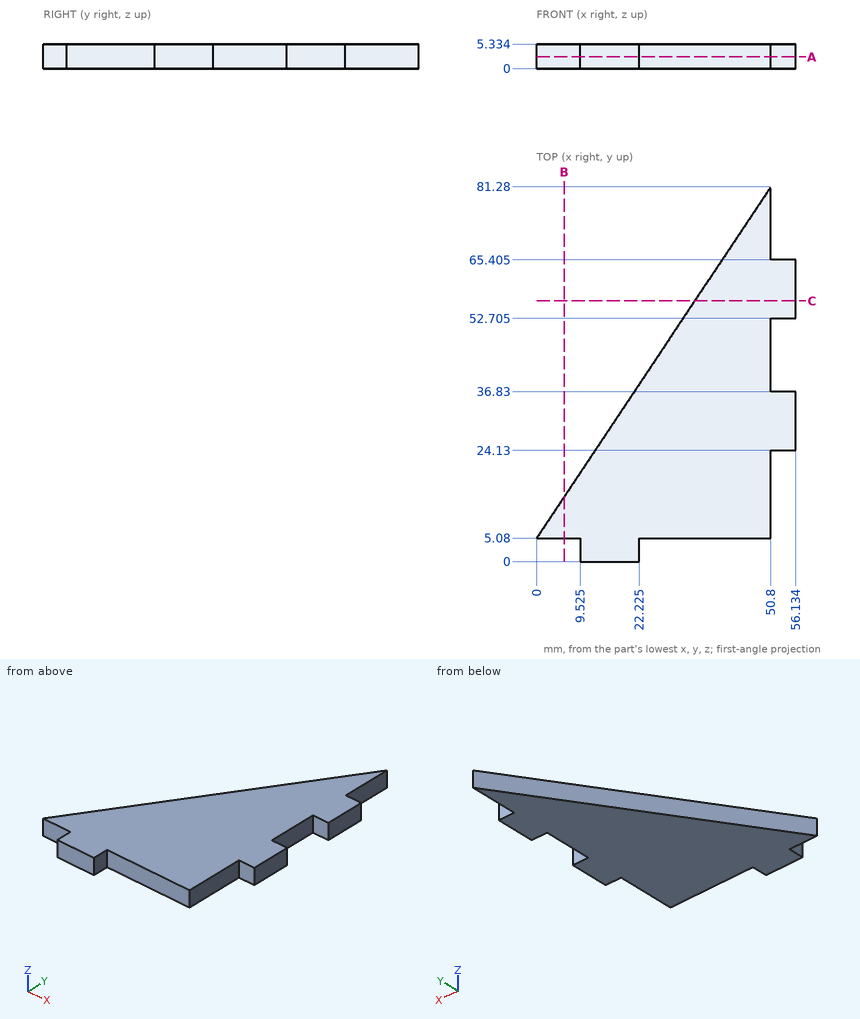
The drawing under review shows one solid part. Ordinate dimensions are in mm from its lowest x, y, z. Give positions to 0.01 mm unless a question says otherwise; leave off trailing zeros. Loops run counter-clockwise (first coordinate to the right, second up) from the corner with the lowest first, then second, coordinate; pieces in that order, holes last. Notation, with made-up numbers: M 83,23 L 101,23 A23 cw 101,33 Z; hole C 79,-2 d7. An arc over 180 degrees is marked long. One line per item, written item: value. Start each with the question number.
Q1. Add section B-B (x = 6). Give the boundary of the cut face in (y, z).
Q2. Add section C-C (y = 56.5). Give the boundary of the cut face in (x, z).
Q3. Add section A-A (z = 2.55). Give the boundary of the cut face in (x, y) (3 decimals), and give its area (3 significant figures).
Q4. For L1, parallel to Y at x = 15.5, z = 3.8; L2, parallel to Y at x = 18, z = 4.4; L3, parallel to X at y = 16, z = 2.3, list the stretches that pass through material, from the lowest coordinate up.
Q5. Clearance check with flat-ended pins moving along their axes: pin 1 Ø2.5 at (x, z) = (53, 2) entering from -Y; pin 2 Ø1.5 at (y, z) = (2.5, 1.5) entering from +X (3 decimals); pin 3 Ø1 at (x, z) = (49, 1.5) entering from -Y. State where each tip first meets the part, or that it passes through.
Reply:
1. outline: M 5.08,0 L 14.08,0 L 14.08,5.33 L 5.08,5.33 Z
2. outline: M 34.28,0 L 56.13,0 L 56.13,5.33 L 34.28,5.33 Z
3. outline: M 0,5.08 L 9.525,5.08 L 9.525,0 L 22.225,0 L 22.225,5.08 L 50.8,5.08 L 50.8,24.13 L 56.134,24.13 L 56.134,36.83 L 50.8,36.83 L 50.8,52.705 L 56.134,52.705 L 56.134,65.405 L 50.8,65.405 L 50.8,81.28 Z
3. area: 2,140 mm²
4. L1: 0 to 28.33
4. L2: 0 to 32.08
4. L3: 7.28 to 50.8
5. pin 1: y = 24.13
5. pin 2: x = 22.225
5. pin 3: y = 5.08
